```python
from build123d import *

# Parameters (mm, degrees)
BOSS_EXTRU_1_DEPTH         = 37.5
CONG_1_R                   = 1
CONG_2_R                   = 1
ENL_V_MAT_EXTRU_1_DEPTH    = 106
CONG_3_R                   = 3
CONG_4_R                   = 3
R_P_TITION_LIN_AIRE2_COUNT = 3
R_P_TITION_LIN_AIRE2_PITCH = 30
CONG_5_R                   = 1


with BuildPart() as part:
    # Esquisse1 → Boss.-Extru.1 (new body, symmetric)
    with BuildSketch(Plane.XY):
        Polygon((50, 0), (50, 5), (-50, 5), (-50, -100), (-45, -100), (-45, 0), align=None)
    extrude(amount=BOSS_EXTRU_1_DEPTH, both=True)

    # Congé1
    cong_1_edges = [part.edges().sort_by_distance(p)[0] for p in [
        (-50, 5, 0),
    ]]
    fillet(cong_1_edges, radius=CONG_1_R)

    # Congé2
    cong_2_edges = [part.edges().sort_by_distance(p)[0] for p in [
        (-45, 0, 0),
    ]]
    fillet(cong_2_edges, radius=CONG_2_R)

    # Esquisse2 → Enlèv. mat.-Extru.1 (cut, through all)
    with BuildSketch(Plane(origin=(0, 5, 0), x_dir=(1, 0, 0), z_dir=(0, 1, 0))):
        with BuildLine():
            Line((13.264657274, 34.025964314), (42.574958683, 14.047069667))
            ThreePointArc((42.574958683, 14.047069667), (50, 0), (42.574958683, -14.047069667))
            Line((42.574958683, -14.047069667), (13.264657274, -34.025964314))
            ThreePointArc((13.264657274, -34.025964314), (7.894095084, -36.611767138), (2, -37.5))
            Line((2, -37.5), (2, -49.357406445))
            Line((2, -49.357406445), (93.230488108, -49.357406445))
            Line((93.230488108, -49.357406445), (93.230488108, 49.357406445))
            Line((93.230488108, 49.357406445), (2, 49.357406445))
            Line((2, 49.357406445), (2, 37.5))
            ThreePointArc((2, 37.5), (7.894095084, 36.611767138), (13.264657274, 34.025964314))
        make_face()
    extrude(amount=-ENL_V_MAT_EXTRU_1_DEPTH, mode=Mode.SUBTRACT)

    # Congé3
    cong_3_edges = [part.edges().sort_by_distance(p)[0] for p in [
        (-47.5, -100, -37.5),
    ]]
    fillet(cong_3_edges, radius=CONG_3_R)

    # Congé4
    cong_4_edges = [part.edges().sort_by_distance(p)[0] for p in [
        (-47.5, -100, 37.5),
    ]]
    fillet(cong_4_edges, radius=CONG_4_R)

    # Esquisse5 → Enlèvement de matière-Révolution2 (revolve, cut)
    with BuildSketch(Plane.XY, mode=Mode.PRIVATE) as enl_vement_de_mati_re_r_volution2_sk:
        Polygon((-44, -87), (-44, -83.75), (-46.25, -83.75), (-50, -80), (-50, -87), align=None)
    enl_vement_de_mati_re_r_volution2 = revolve(enl_vement_de_mati_re_r_volution2_sk.sketch.rotate(Axis((-72.134969263, -87, 0), (1, 0, 0)), 90), axis=Axis((-72.134969263, -87, 0), (1, 0, 0)), mode=Mode.SUBTRACT)  # turned: the seam where the file's is

    # Répétition linéaire2: Enlèvement de matière-Révolution2 ×3
    with Locations(*[(0, i * R_P_TITION_LIN_AIRE2_PITCH, 0) for i in range(1, R_P_TITION_LIN_AIRE2_COUNT)]):
        add(enl_vement_de_mati_re_r_volution2, mode=Mode.SUBTRACT)

    # Congé5
    cong_5_edges = [part.edges().sort_by_distance(p)[0] for p in [
        (-50, -46.5, -37.5),
        (-50, -46.5, 37.5),
        (-49.707106781, 4.707106781, -37.5),
        (-49.707106781, 4.707106781, 37.5),
        (-21, 0, -37.5),
        (-21, 0, 37.5),
        (-44.707106781, -0.292893219, 37.5),
        (-44.707106781, -0.292893219, -37.5),
        (-23.5, 5, -37.5),
        (-23.5, 5, 37.5),
        (27.919807978, 0, 24.03651699),
        (50, 0, 0),
        (27.919807978, 0, -24.03651699),
        (7.894095084, 0, 36.611767138),
        (7.894095084, 0, -36.611767138),
        (50, 5, 0),
        (7.894095084, 5, -36.611767138),
        (27.919807978, 5, -24.03651699),
        (27.919807978, 5, 24.03651699),
        (7.894095084, 5, 36.611767138),
        (-45, -49, -37.5),
        (-45, -99.121320344, -36.621320344),
        (-50, -99.121320344, -36.621320344),
        (-45, -49, 37.5),
        (-50, -100, 0),
        (-45, -100, 0),
        (-50, -99.121320344, 36.621320344),
        (-45, -99.121320344, 36.621320344),
    ]]
    fillet(cong_5_edges, radius=CONG_5_R)

    # Esquisse6 → Enlèvement de matière-Révolution3 (revolve, cut)
    with BuildSketch(Plane.XY):
        Polygon((38, 6), (35, 6), (35, 4), (30, -1), (38, -1), align=None)
    revolve(axis=Axis((38, 8.257594869, 0), (0, -1, 0)), mode=Mode.SUBTRACT)

    # Esquisse10 → Enlèvement de matière-Révolution5 (revolve, cut)
    with BuildSketch(Plane.XY.offset(28.5)):
        Polygon((4, 6), (1, 6), (1, 4), (-4, -1), (4, -1), align=None)
    enl_vement_de_mati_re_r_volution5 = revolve(axis=Axis((4, 7.732158055, 28.5), (0, -1, 0)), mode=Mode.SUBTRACT)

    # Symétrie1: Enlèvement de matière-Révolution5 across plane
    add(enl_vement_de_mati_re_r_volution5.mirror(Plane.XY), mode=Mode.SUBTRACT)


solid = part.part
```
Design review of the part built by this model. Coordinates are the model's own, in mm. A direction names the side the tool comes from. Coordinates: 2 decimals unless noted, no trailing zeros. Loops run counter-clockwise (first coordinate to the right, second up) from the corner with the lowest first, then second, coordinate; pieces in that order, holes last.
Q1. To check wall thickness, follow line 1 (Y direction, x = -45.95, z = 0); line 2 (X direction, y = -7, z = -18.5); line 3 (Z direction, x = 4, y = 4). State the ranges of each line that lie inside material, in increasing order.
Reported:
line 1: y = -100 to -90.25, -83.75 to -60.25, -53.75 to -30.25, -23.75 to 5
line 2: x = -50 to -45
line 3: z = -37.4 to -31.5, -25.5 to 25.5, 31.5 to 37.4
Q2. We need section C-C on z = 0. State how many separate pieces and enclosed holes the cut face has, and give its area (3 significant figures).
Reported:
separate pieces: 5
enclosed holes: 0
area: 813 mm2
Q3. We need section B-B on x = -34.5. State the section outline as (y, z) points.
Reported:
outline: (0, -36.5) arc R1 ccw to (1, -37.5) - (4, -37.5) arc R1 ccw to (5, -36.5) - (5, 36.5) arc R1 ccw to (4, 37.5) - (1, 37.5) arc R1 ccw to (0, 36.5) - close
Q4. The part is to be moulded in two halves that separate along X. For faces 1 (the face through (1.23, 4.49, 29.65)), 2 (the face through (-47.48, -99.1, -36.64)), 3 (the face through (-46.485, -59.355, -2.568)), say which applies: +X half, -X half, draft (parallel to the pull), parting line (faces both ways), or undercut.
Reported:
face 1: undercut
face 2: draft
face 3: -X half
Q5. For pin 1 (3 mm diameter, centred on x = -34.5, z = 17, fed in from -Y); pin 2 (7.5 mm diameter, centred on y = -27, z = 0, fed in from -X); pin 3 (7 mm diameter, centred on x = 4, z = -28.5, fed in from -Y); pin 4 (5 mm diameter, centred on x = 38, z = 0, fed in from -Y), all flat-tipped, find the tip position at first contact; note any pin that passes through.
Reported:
pin 1: stops at y = 0
pin 2: stops at x = -46.75
pin 3: stops at y = 3.5
pin 4: passes through
Q6. Tool access review of faces 4 (the face through (27.96, 0.3, -23.66)), 5 (the face through (-45, -51, 1)): name each direction out of +Z, -Z, +X, -X, +Y, -Y from which nothing blocks a thin tool from reaching the whole face with its end or side.
Reported:
face 4: -Z, +X, -Y
face 5: +Z, -Z, +X, -Y
Q7. We need section A-A on y = -57. State the section outline as (x, z) points, and give its area (3 significant figures).
Reported:
outline: (-50, -36.5) arc R1 ccw to (-49, -37.5) - (-46, -37.5) arc R1 ccw to (-45, -36.5) - (-45, -3.25) - (-46.25, -3.25) - (-50, -7) - close; (-50, 7) - (-46.25, 3.25) - (-45, 3.25) - (-45, 36.5) arc R1 ccw to (-46, 37.5) - (-49, 37.5) arc R1 ccw to (-50, 36.5) - close
area: 328 mm2
